```python
from build123d import *

# Parameters (mm, degrees)
PLAIN_BEARING_RETAINER_SKETCH_R        = 15.9
PLAIN_BEARING_RETAINER_EXTRUSION_DEPTH = 44.8
RETAINER_START                         = -3
RETAINER_WALL_EXTRUDE_OUTLINE_R        = 11
RETAINER_WALL_EXTRUDE_DEPTH            = 3
M5_CLEARANCE_HOLE1_D                   = 5.5
CIRPATTERN1_COUNT                      = 5
FILLET1_R                              = 3
F_6_4MM_M5_INSERT_HOLE_D               = 6.4
F_6_4MM_M5_INSERT_HOLE_DEPTH           = 10
F_6_4MM_M5_INSERT_HOLE_TIP             = 1.922753981


# Read off the part's stored shape, not the designer's step: Retainer Wall Extrude
with BuildPart() as part:
    # Plain Bearing Retainer Sketch → Plain Bearing Retainer Extrusion (new body)
    with BuildSketch(Plane.XY):
        with BuildLine():
            ThreePointArc((32.9, 0), (-9.910302975, 31.371896579), (-26.929537686, -18.9))
            Line((-26.929537686, -18.9), (26.929537686, -18.9))
            ThreePointArc((26.929537686, -18.9), (31.371896579, -9.910302975), (32.9, 0))
        make_face()
        Circle(PLAIN_BEARING_RETAINER_SKETCH_R, mode=Mode.SUBTRACT)
    extrude(amount=PLAIN_BEARING_RETAINER_EXTRUSION_DEPTH)

    # Retainer Wall Extrude outline → Retainer Wall Extrude (add)
    with BuildSketch(Plane.XY.offset(RETAINER_START)):
        with BuildLine():
            Line((-26.929537686, -18.9), (26.929537686, -18.9))
            ThreePointArc((26.929537686, -18.9), (0, 32.9), (-26.929537686, -18.9))
        make_face()
        Circle(RETAINER_WALL_EXTRUDE_OUTLINE_R, mode=Mode.SUBTRACT)
    extrude(amount=RETAINER_WALL_EXTRUDE_DEPTH)

    # M5 Clearance Hole1 (through all)
    with Locations(Plane.XY.offset(44.8)):
        with Locations((13.460282277, 18.526489171)):
            m5_clearance_hole1 = Hole(M5_CLEARANCE_HOLE1_D / 2)

    # CirPattern1: M5 Clearance Hole1 ×5 about axis, 1 skipped
    cirpattern1_axis = Axis((0, 0, 0), (0, 0, -1))
    add([m5_clearance_hole1.rotate(cirpattern1_axis, i * 360 / CIRPATTERN1_COUNT) for i in range(1, CIRPATTERN1_COUNT) if i not in (2,)], mode=Mode.SUBTRACT)

    # Fillet1
    fillet1_edges = [part.edges().sort_by_distance(p)[0] for p in [
        (-26.929537686, -18.9, 22.4),
        (26.929537686, -18.9, 22.4),
    ]]
    fillet(fillet1_edges, radius=FILLET1_R)

    # Ø6.4mm M5 Insert Hole
    with Locations(Plane(origin=(0, 0, -3), x_dir=(-1, 0, 0), z_dir=(0, 0, -1))):
        with Locations((-13.460282277, 18.526489171), (-21.779194223, -7.076489171), (21.779194223, -7.076489171), (13.460282277, 18.526489171)):
            Hole(F_6_4MM_M5_INSERT_HOLE_D / 2, depth=F_6_4MM_M5_INSERT_HOLE_DEPTH)
            with Locations((0, 0, -(F_6_4MM_M5_INSERT_HOLE_DEPTH + F_6_4MM_M5_INSERT_HOLE_TIP / 2))):  # 118° drill point
                Cone(0, F_6_4MM_M5_INSERT_HOLE_D / 2, F_6_4MM_M5_INSERT_HOLE_TIP, mode=Mode.SUBTRACT)


solid = part.part
```
Build history of the part. All positions in model axes, mm. A direction names the side the tool comes from. Round coordinates to 2 decimals unless told otherwise and drop trailing zeros. Write each loop counter-clockwise with the first axis right and the second up, starting at its lowest first coordinate (ties: lowest second). Pieces come first, ordered by that corner, then holes.
1) Drill centre lines: probe 1 along X at (y, z) = (-9.5, 9.5); probe 2 along Y at (x, z) = (0, 32); probe 3 along Y at (x, z) = (12.5, 6). Where is each one in solid material? Low to high.
2) Pin check, flat tips, straight feed: pin 1 (8 mm diameter, centred on x = -20, z = 37, fed in from +Y); pin 2 (8 mm diameter, centred on x = 0, z = 15, fed in from +Y); pin 3 (1.5 mm diameter, centred on y = 0.5, z = 28, fed in from -X); pin 4 (6 mm diameter, centred on x = -21.78, y = -7.08, fed in from -Z). Stop position of each tip, or through.
3) Band-saw the part on A-A, the plane x = 0. List the corners of the cut face in (y, z), and give its area (3 significant figures).
4) Band-saw the part on B-B, the plane z = 3. List the corners of the cut face in (x, y), and give its area (3 significant figures).
5) Mould opens along Y. For faces 1 (the flat face through (0, -18.9, 21)), 2 (the flat face through (0, 13, -3)), 3 (the cylindrical face through (-2.38, -10.74, -1.52)) say: +Y half, -Y half, draft (parallel to the pull), parting line (faces both ways), or undercut.
6) Band-saw the part on D-D, the plane x = 8.5. List the corners of the cut face in (y, z), and give its area (3 significant figures).
7) 3-axis set-ups, long thin cutter, end or side, ignore diameter. For faces 4 (the cylindrical face through (-11.98, 15.69, 2.07)), 5 (the cylindrical face through (26.75, -18.54, 21.23)), 6 (the flat face through (3, 11, 0)): which of +Z, -Z, +X, -X, +Y, -Y reach the whole face in a straight line?
8) Band-saw the part on C-C, the plane y = -13.5. List the corners of the cut face in (x, z).
Ans:
1. probe 1: x = -31.5 to -23.08, -20.48 to -12.75, 12.75 to 20.48, 23.08 to 31.5
1. probe 2: y = -18.9 to -15.9, 15.9 to 32.9
1. probe 3: y = -18.9 to -9.83, 9.83 to 15.47, 21.58 to 30.43
2. pin 1: stops at y = 28.75
2. pin 2: stops at y = 32.9
2. pin 3: stops at x = -32.9
2. pin 4: stops at z = 7.12
3. outline: (-18.9, -3) - (-11, -3) - (-11, 0) - (-15.9, 0) - (-15.9, 44.8) - (-18.9, 44.8) - close; (11, -3) - (32.9, -3) - (32.9, 44.8) - (15.9, 44.8) - (15.9, 0) - (11, 0) - close
3. area: 985 mm2
4. outline: (-27.86, -17.5) arc R3 ccw to (-25.32, -18.9) - (25.32, -18.9) arc R3 ccw to (27.86, -17.5) arc R32.9 ccw (long way) to start; hole circle Ø6.4 at (-21.78, -7.08); hole circle Ø6.4 at (-13.46, 18.53); hole circle Ø31.8 at (0, 0); hole circle Ø6.4 at (13.46, 18.53); hole circle Ø6.4 at (21.78, -7.08)
4. area: 1,950 mm2
5. face 1: -Y half
5. face 2: draft
5. face 3: undercut
6. outline: (-18.9, -3) - (-6.98, -3) - (-6.98, 0) - (-13.44, 0) - (-13.44, 44.8) - (-18.9, 44.8) - close; (6.98, -3) - (31.78, -3) - (31.78, 44.8) - (13.44, 44.8) - (13.44, 0) - (6.98, 0) - close
6. area: 1,180 mm2
7. face 4: -Z
7. face 5: +Z, -Z, +X, -Y
7. face 6: +Z
8. outline: (-30, -3) - (30, -3) - (30, 44.8) - (8.4, 44.8) - (8.4, 0) - (-8.4, 0) - (-8.4, 44.8) - (-30, 44.8) - close
